```python
from build123d import *

# Parameters (mm, degrees)
BOSS_EXTRUDE1_DEPTH = 30
FILLET3_R           = 20
FILLET4_R           = 21.25
FILLET5_R           = 1.25


with BuildPart() as part:
    # Sketch1 → Boss-Extrude1 (new body)
    with BuildSketch(Plane.XY):
        Polygon((-67.5, 15), (-57.5, 15), (-57.5, 67.5), (57.5, 67.5), (57.5, 15), (67.5, 15), (67.5, 20), (60, 20), (60, 70), (-60, 70), (-60, 20), (-67.5, 20), align=None)
    extrude(amount=BOSS_EXTRUDE1_DEPTH)

    # Fillet3
    fillet3_edges = [part.edges().sort_by_distance(p)[0] for p in [
        (57.5, 67.5, 15),
        (-57.5, 67.5, 15),
    ]]
    fillet(fillet3_edges, radius=FILLET3_R)

    # Fillet4
    fillet4_edges = [part.edges().sort_by_distance(p)[0] for p in [
        (-60, 70, 15),
        (60, 70, 15),
    ]]
    fillet(fillet4_edges, radius=FILLET4_R)

    # Fillet5
    fillet5_edges = [part.edges().sort_by_distance(p)[0] for p in [
        (-57.5, 31.25, 0),
        (60, 34.375, 0),
        (60, 34.375, 30),
        (57.5, 31.25, 0),
        (57.5, 31.25, 30),
        (0, 67.5, 0),
        (0, 67.5, 30),
        (51.642135624, 61.642135624, 0),
        (51.642135624, 61.642135624, 30),
        (-51.642135624, 61.642135624, 0),
        (-51.642135624, 61.642135624, 30),
        (-57.5, 31.25, 30),
        (0, 70, 0),
        (0, 70, 30),
        (-60, 34.375, 0),
        (-53.7760191, 63.7760191, 0),
        (53.7760191, 63.7760191, 0),
        (-60, 34.375, 30),
        (-53.7760191, 63.7760191, 30),
        (53.7760191, 63.7760191, 30),
    ]]
    fillet(fillet5_edges, radius=FILLET5_R - 0.0001)  # a hair under: the kernel refuses the full size


solid = part.part
```
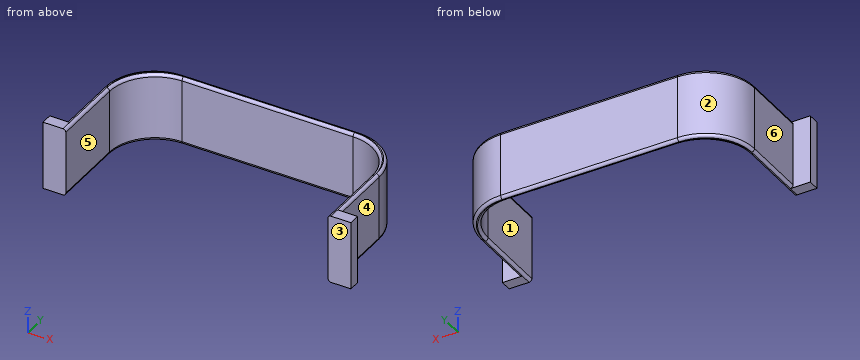
Read the model definition and answer for the solid it produces. Units are mm, in the model's axes. Face numbers are marked on the shaded views. A direction names the side the tool comes from. Round coordinates to 2 decimals unless told otherwise and drop trailing zeros. Loops run counter-clockwise (first coordinate to the right, second up) from the corner with the lowest first, then second, coordinate; pieces in that order, holes last. Notation, with made-up numbers: (-31.5, 43.5) -> (8.5, 43.5) arc R10 ccw to (8.5, 54.5) -> close; hole circle Ø11 at (50, 54). An arc over 180 degrees is marked (long way). One line per item, written item: value.
1) For the marked faces 4, 5 and 6, determine the directions among +Z, -Z, +X, -X, +Y, -Y from which every point of the face is accessible in a straight line to the end or side of a thin tool.
Answer list:
face 4: +Z, -Z, +X, +Y
face 5: +Z, -Z, -Y
face 6: +Z, -Z, -X, +Y
2) Consider L1, parallel to X at y = 21.5, z = 10.5; L2, parallel to Y at x = 17.5, z = 24; L3, parallel to X at y = 64.5, z = 4. Determine where each line is inside the solid, lowest interval first. Write a range as [from, to].
Answer list:
L1: x = [-60, -57.5], [57.5, 60]
L2: y = [67.5, 70]
L3: x = [-53.02, -48.04], [48.04, 53.02]
3) Flat-ended cylindrical pins translate along their axes: P1, Ø5, axis at x = -22, z = 14.5, coming from the -Y side; P2, Ø12, axis at y = 37, z = 17, coming from the -X side; P3, Ø8.5, axis at y = 33.5, z = 20.5, coming from the +X side. Find the tip coordinate at first contact, or state that the pin passes through.
Answer list:
P1: stops at y = 67.5
P2: stops at x = -60
P3: stops at x = 60
4) A cutting plane is placed at C-C (z = 12). Determine the outline of the cut face in (x, y), and give its area (3 significant figures).
Answer list:
outline: (-67.5, 15) -> (-57.5, 15) -> (-57.5, 47.5) arc R20 cw to (-37.5, 67.5) -> (37.5, 67.5) arc R20 cw to (57.5, 47.5) -> (57.5, 15) -> (67.5, 15) -> (67.5, 20) -> (60, 20) -> (60, 48.75) arc R21.25 ccw to (38.75, 70) -> (-38.75, 70) arc R21.25 ccw to (-60, 48.75) -> (-60, 20) -> (-67.5, 20) -> close
area: 615 mm²
5) The mould has two halves that part along X. Classify the marked faces 1, 2 and 3: pulls with the +X half, pulls with the -X half, needs draft (parallel to the pull), parting line crosses it, or undercut.
Answer list:
face 1: undercut
face 2: pulls with the -X half
face 3: needs draft
